Work out the finished part from the listing and answer in its coordinate system (mm). A direction names the side the tool comes from. Coordinates: 2 decimals unless noted, no trailing zeros. Loops run counter-clockwise (first coordinate to the right, second up) from the corner with the lowest first, then second, coordinate; pieces in that order, holes last. Notation, with made-up numbers: (46, 89) - (90, 89) arc R5 cw to (90, 97) - close; hole circle Ø6 at (-29, 67). An arc over 180 degrees is marked (long way). Write each question's results on one line, items separated by ' | '. Start each with the question number.
1. Determine the mould class of faces 3 (the cylindrical face through (2.296, -9.86, 83.972)), 4 (the flat face through (-9, -20, 45)) for opening direction X: released by +X, released by -X, zero draft, split by the parting line, or undercut.
2. Which of the six approach directions +Z, -Z, +X, -X, +Y, -Y give full straight-line access (tool end or side, diameter ignored) to faces 1 (the cylindrical face through (-12.92, -9.86, 33.973)), 2 (the cylindrical face through (-13.2, -9.86, -163.566))?
3. A cutting plane is placed at B-B on x = -685.5. Determine the outline of the cut face in (y, z), then the cut area to 3 significant figures.
4. Each of these flat-tipped pins is pushed along its axis until it touches: P1, Ø1, axis at y = -11, z = 93, coming from the +X side; P2, Ø12, axis at y = -8, z = 35.5, coming from the -X side; P3, Ø1, axis at x = 301, y = -6, coming from the +Z side. Where does it stop, or does it pass through?
5. Find the intervals of material crossed by line 1 along X through (y, z) = (-4.5, 0); line 2 along Z through (x, y) = (8, -5.25); line 3 along X through (y, z) = (-9.25, -74), in increasing order. Write a range as [from, to].
6. A cutting plane is placed at A-A on z = 0. Determine the outline of the cut face in (x, y).
7. A cutting plane is placed at C-C on y = -15.5. Determine the outline of the cut face in (x, z).
8. A cutting plane is placed at D-D on z = 98. Determine the outline of the cut face in (x, y).
from build123d import *

# Parameters (mm, degrees)
F1_DEPTH = 20


with BuildPart() as f1:
    # F0 (on Front) → F1 (new body)
    with BuildSketch(Plane.XZ):
        with BuildLine():
            ThreePointArc((515.887824, 184.479399), (-5.178885, 83.952454), (-526.245594, 184.479399))
            ThreePointArc((-526.245594, 184.479399), (-797.205456, 26.06358), (-576.7568, -197.358015))
            ThreePointArc((-576.7568, -197.358015), (-5.178885, -163.559701), (566.399031, -197.358015))
            ThreePointArc((566.399031, -197.358015), (786.847687, 26.06358), (515.887824, 184.479399))
        make_face()
        with BuildLine():
            ThreePointArc((-582.649356, -147.706451), (-747.637277, 19.506473), (-544.845819, 138.067852))
            ThreePointArc((-544.845819, 138.067852), (-5.178885, 33.952454), (534.488049, 138.067852))
            ThreePointArc((534.488049, 138.067852), (737.279508, 19.506473), (572.291587, -147.706451))
            ThreePointArc((572.291587, -147.706451), (-5.178885, -113.559701), (-582.649356, -147.706451))
        make_face(mode=Mode.SUBTRACT)
    extrude(amount=F1_DEPTH)


solid = f1.part
Values:
1) face 3: undercut | face 4: zero draft
2) face 1: +Y, -Y | face 2: -Z, +Y, -Y
3) outline: (-20, -179.5) - (0, -179.5) - (0, -121.84) - (-20, -121.84) - close; (-20, 121.84) - (0, 121.84) - (0, 179.5) - (-20, 179.5) - close | area: 2,310 mm^2
4) P1: x = 765.73 | P2: x = -796.72 | P3: z = 117.94
5) line 1: [-798.92, -748.92], [738.56, 788.56] | line 2: [-163.58, -113.58], [34.01, 84.01] | line 3: [-784.63, -729.21], [718.85, 774.27]
6) outline: (-798.92, -20) - (-748.92, -20) - (-748.92, 0) - (-798.92, 0) - close; (738.56, -20) - (788.56, -20) - (788.56, 0) - (738.56, 0) - close
7) outline: (-576.76, -197.36) arc R4850 cw to (566.4, -197.36) arc R198.74 ccw (long way) to (515.89, 184.48) arc R1400.7 cw to (-526.25, 184.48) arc R198.74 ccw (long way) to start; hole (-582.65, -147.71) arc R4900 cw to (572.29, -147.71) arc R148.74 ccw (long way) to (534.49, 138.07) arc R1450.7 cw to (-544.85, 138.07) arc R148.74 ccw (long way) to start
8) outline: (-773.08, -20) - (-712.07, -20) - (-712.07, 0) - (-773.08, 0) - close; (-431.47, -20) - (-203.06, -20) - (-203.06, 0) - (-431.47, 0) - close; (192.7, -20) - (421.11, -20) - (421.11, 0) - (192.7, 0) - close; (701.72, -20) - (762.72, -20) - (762.72, 0) - (701.72, 0) - close
